```python
from build123d import *

# Parameters (mm, degrees)
SKETCH1_R            = 19.85
SKETCH1_R_2          = 18.78
BOSS_EXTRUDE3_DEPTH  = 7.95
SKETCH2_R            = 18.78
BOSS_EXTRUDE5_DEPTH  = 1.5
SKETCH4_R            = 12.5
BOSS_EXTRUDE6_DEPTH  = 16.31
SKETCH5_R            = 2.15
SKETCH5_W            = 4.3
SKETCH5_H            = 2.15
CUT_EXTRUDE2_DEPTH   = 16.31
SKETCH6_R            = 11.597360911
CUT_EXTRUDE3_DEPTH   = 14.809999892
SKETCH12_R           = 3.4
SKETCH12_W           = 6.8
SKETCH12_H           = 3.4
BOSS_EXTRUDE8_DEPTH  = 24.969999892
SKETCH5_6_R          = 2.15
SKETCH5_6_W          = 4.3
SKETCH5_6_H          = 2.15
CUT_EXTRUDE5_DEPTH   = 24.969999892
CUT_EXTRUDE6_START   = -14.81
SKETCH14_R           = 15.219310499
SKETCH14_R_2         = 12.5
CUT_EXTRUDE6_DEPTH   = 14.81
SKETCH17_W           = 6.8
SKETCH17_H           = 2.662223843
CUT_EXTRUDE7_DEPTH   = 16.587999892
SKETCH18_R           = 3.4
SKETCH18_R_2         = 2.15
BOSS_EXTRUDE10_DEPTH = 14
SKETCH19_R           = 5.618160511
SKETCH19_R_2         = 3.4
CUT_EXTRUDE8_DEPTH   = 14


with BuildPart() as part:
    # Sketch1 → Boss-Extrude3 (new body)
    with BuildSketch(Plane(origin=(0, 0, 0), x_dir=(1, 0, 0), z_dir=(0, 1, 0))):
        Circle(SKETCH1_R)
        Circle(SKETCH1_R_2, mode=Mode.SUBTRACT)
    extrude(amount=BOSS_EXTRUDE3_DEPTH)

    # Sketch2 → Boss-Extrude5 (add)
    with BuildSketch(Plane.XZ):
        Circle(SKETCH2_R)
    extrude(amount=-BOSS_EXTRUDE5_DEPTH)


with BuildPart() as body_2:
    # Sketch4 → Boss-Extrude6 (new body)
    with BuildSketch(Plane.XZ):
        Circle(SKETCH4_R)
    extrude(amount=-BOSS_EXTRUDE6_DEPTH)


with BuildPart() as cut_extrude2_tool:
    # Sketch5 → Cut-Extrude2 (new body)
    with BuildSketch(Plane(origin=(0, 16.31, 0), x_dir=(1, 0, 0), z_dir=(0, 1, 0))):
        with Locations((0, 10.35)):
            Circle(SKETCH5_R)
        with Locations((0, 11.425)):
            Rectangle(SKETCH5_W, SKETCH5_H)
    extrude(amount=-CUT_EXTRUDE2_DEPTH)


with BuildPart() as part_1:
    add(part.part)

    # Cut-Extrude2: cut by cut_extrude2_tool
    add(cut_extrude2_tool.part, mode=Mode.SUBTRACT)


with BuildPart() as body_2_1:
    add(body_2.part)

    # Cut-Extrude2: cut by cut_extrude2_tool
    add(cut_extrude2_tool.part, mode=Mode.SUBTRACT)


with BuildPart() as cut_extrude3_tool:
    # Sketch6 → Cut-Extrude3 (new body)
    with BuildSketch(Plane.XZ):
        Circle(SKETCH6_R)
    extrude(amount=-CUT_EXTRUDE3_DEPTH)


with BuildPart() as part_2:
    add(part_1.part)

    # Cut-Extrude3: cut by cut_extrude3_tool
    add(cut_extrude3_tool.part, mode=Mode.SUBTRACT)



with BuildPart() as body_2_2:
    add(body_2_1.part)

    # Cut-Extrude3: cut by cut_extrude3_tool
    add(cut_extrude3_tool.part, mode=Mode.SUBTRACT)


with BuildPart() as part_3:
    add(part_2.part)

    add(body_2_2.part)  # Boss-Extrude8 merges body 2
    # Sketch12 → Boss-Extrude8 (add)
    with BuildSketch(Plane(origin=(0, 16.31, 0), x_dir=(1, 0, 0), z_dir=(0, 1, 0))):
        with Locations((0, 10.35)):
            Circle(SKETCH12_R)
        with Locations((0, 12.05)):
            Rectangle(SKETCH12_W, SKETCH12_H)
    extrude(amount=-BOSS_EXTRUDE8_DEPTH)

    # Sketch5<6> → Cut-Extrude5 (cut)
    with BuildSketch(Plane(origin=(0, 16.31, 0), x_dir=(1, 0, 0), z_dir=(0, 1, 0))):
        with Locations((0, 10.35)):
            Circle(SKETCH5_6_R)
        with Locations((0, 11.425)):
            Rectangle(SKETCH5_6_W, SKETCH5_6_H)
    extrude(amount=-CUT_EXTRUDE5_DEPTH, mode=Mode.SUBTRACT)

    # Sketch14 → Cut-Extrude6 (cut)
    with BuildSketch(Plane(origin=(0, 16.31, 0), x_dir=(1, 0, 0), z_dir=(0, 1, 0)).offset(CUT_EXTRUDE6_START)):
        Circle(SKETCH14_R)
        Circle(SKETCH14_R_2, mode=Mode.SUBTRACT)
    extrude(amount=CUT_EXTRUDE6_DEPTH, mode=Mode.SUBTRACT)

    # Sketch17 → Cut-Extrude7 (cut)
    with BuildSketch(Plane.XZ):
        with Locations((0, -12.418888079)):
            Rectangle(SKETCH17_W, SKETCH17_H)
    extrude(amount=CUT_EXTRUDE7_DEPTH, mode=Mode.SUBTRACT)

    # Sketch18 → Boss-Extrude10 (add)
    with BuildSketch(Plane.XZ):
        with Locations((0, -10.35)):
            Circle(SKETCH18_R)
        with Locations((0, -10.35)):
            Circle(SKETCH18_R_2, mode=Mode.SUBTRACT)
    extrude(amount=BOSS_EXTRUDE10_DEPTH)

    # Sketch19 → Cut-Extrude8 (cut)
    with BuildSketch(Plane.XZ):
        with Locations((0, -10.35)):
            Circle(SKETCH19_R)
        with Locations((0, -10.35)):
            Circle(SKETCH19_R_2, mode=Mode.SUBTRACT)
    extrude(amount=CUT_EXTRUDE8_DEPTH, mode=Mode.SUBTRACT)


solid = part_3.part
```
Model file for the job. Use its own axes, mm. A direction names the side the tool comes from. Coordinates: 2 decimals unless noted, no trailing zeros. Write each loop counter-clockwise with the first axis right and the second up, starting at its lowest first coordinate (ties: lowest second). Pieces come first, ordered by that corner, then holes. Notation, with made-up numbers: (33.25, 12.25) - (54.25, 12.25) arc R18 cw to (54.25, 25.25) - close; hole circle Ø2 at (49.25, 22.25). An arc over 180 degrees is marked (long way). Use a Markdown table: item, result. Add a question column.
Item 1: Drop flat-ended pins along their axis: pin 1 (1.1 mm diameter, centred on x = -1, z = -11, fed in from +Y); pin 2 (4 mm diameter, centred on x = 12.5, y = -1.5, fed in from +Z); pin 3 (6 mm diameter, centred on x = 5.5, y = 6, fed in from +Z); pin 4 (18 mm diameter, centred on x = -1.5, z = 5, fed in from -Y). Give the stop position or say it passes through.
Item 2: Band-saw the part on B-B, the plane z = 0. Write the cut outline in (x, y).
Item 3: Band-saw the part on D-D, the plane y = -10. Write the cut outline in (x, z), and give its area (3 significant figures).
Item 4: 3-axis set-ups, long thin cutter, end or side, ignore diameter. For faces 1 (the face through (-15.75, 3.92, 12.08)), 2 (the face through (0, 14.81, 0)), 3 (the face through (0, 1, -12.5)): which of +Z, -Z, +X, -X, +Y, -Y reach the whole face in a straight line?
Item 5: Band-saw the part on A-A, the plane y = 11. Write the cut outline in (x, z), and give its area (3 significant figures).
Item 6: Band-saw the part on C-C, the plane x = -9. Write the cut outline in (y, z).
Item 7: Drill centre lines: line 1 along X through (y, z) = (5.75, 0); line 2 along Z through (x, y) = (0, -6.5); line 3 along Z through (x, y) = (-6.5, 2.5). Where is each one in solid material? Low to high.
A:
| question | item | result |
|---|---|---|
| 1 | pin 1 | passes through |
| 1 | pin 2 | stops at z = 16.4 |
| 1 | pin 3 | stops at z = 19.69 |
| 1 | pin 4 | stops at y = 0 |
| 2 | outline | (-19.85, 0) - (-11.6, 0) - (-11.6, 14.81) - (11.6, 14.81) - (11.6, 0) - (19.85, 0) - (19.85, 7.95) - (18.78, 7.95) - (18.78, 1.5) - (12.5, 1.5) - (12.5, 16.31) - (-12.5, 16.31) - (-12.5, 1.5) - (-18.78, 1.5) - (-18.78, 7.95) - (-19.85, 7.95) - close |
| 3 | outline | circle Ø6.8 at (0, -10.35); hole circle Ø4.3 at (0, -10.35) |
| 3 | area | 21.8 mm² |
| 4 | face 1 | +Y, -Y |
| 4 | face 2 | -Y |
| 4 | face 3 | +Y |
| 5 | outline | (-2.15, -12.31) - (-2.15, -10.35) arc R2.15 cw to (2.15, -10.35) - (2.15, -12.31) arc R12.5 ccw (long way) to start; hole (-3.4, -11.09) - (-3.4, -10.35) arc R3.4 cw to (3.4, -10.35) - (3.4, -11.09) arc R11.6 ccw (long way) to start |
| 5 | area | 77.6 mm² |
| 6 | outline | (0, -17.69) - (7.95, -17.69) - (7.95, -16.48) - (1.5, -16.48) - (1.5, -8.67) - (16.31, -8.67) - (16.31, 8.67) - (1.5, 8.67) - (1.5, 16.48) - (7.95, 16.48) - (7.95, 17.69) - (0, 17.69) - (0, 7.31) - (14.81, 7.31) - (14.81, -7.31) - (0, -7.31) - close |
| 7 | line 1 | x = -19.85 to -18.78, -12.5 to -11.6, 11.6 to 12.5, 18.78 to 19.85 |
| 7 | line 2 | z = -13.75 to -12.5, -8.2 to -6.95 |
| 7 | line 3 | z = -18.76 to -17.62, -10.68 to -9.6, 9.6 to 10.68, 17.62 to 18.76 |
